from build123d import *

# Parameters (mm, degrees)
F2_DEPTH      = 20
F3_W          = 1
F3_H          = 28.1
F4_DEPTH      = 15.101
F4_DEPTH_BACK = 15.101
F5_R          = 2.6
F6_DEPTH      = 15.101
F6_DEPTH_BACK = 15.101
F7_R          = 2.6
F8_DEPTH      = 8
F9_R          = 5
F10_DEPTH     = 3
F11_S5_R      = 5
F11_T6_DEPTH  = 9
F11_S11_R     = 5
F11_T12_DEPTH = 9
F12_R         = 1


# Not quite as in the source:
# - a fillet or chamfer that OpenCascade refuses, or shapes differently, is made with other operations: its cross-section is extruded or revolved along the edge and cut away or added


with BuildPart() as f2:
    # F1 (on Front) → F2 (new body, symmetric)
    with BuildSketch(Plane.XZ):
        Polygon((15.1, 16), (10.1, 16), (10.1, -10.1), (-10.1, -10.1), (-10.1, 16), (-15.1, 16), (-15.1, -18.1), (15.1, -18.1), align=None)
    extrude(amount=F2_DEPTH, both=True)

    # F3 (on Right) → F4 (cut, two sides)
    with BuildSketch(Plane.YZ) as f4_sk:
        with Locations((0, 1.95)):
            Rectangle(F3_W, F3_H)
    extrude(amount=-F4_DEPTH, mode=Mode.SUBTRACT)
    extrude(f4_sk.sketch, amount=F4_DEPTH_BACK, mode=Mode.SUBTRACT)

    # F5 (on Right) → F6 (cut, two sides)
    with BuildSketch(Plane.YZ) as f6_sk:
        with Locations((10, 0)):
            Circle(F5_R)
        with Locations((-10, 0)):
            Circle(F5_R)
    extrude(amount=-F6_DEPTH, mode=Mode.SUBTRACT)
    extrude(f6_sk.sketch, amount=F6_DEPTH_BACK, mode=Mode.SUBTRACT)

    # F7 (on face) → F8 (cut, through all)
    with BuildSketch(Plane(origin=(0, 0, -18.1), x_dir=(1, 0, 0), z_dir=(0, 0, -1))):
        with Locations((0, 10)):
            Circle(F7_R)
        with Locations((0, -10)):
            Circle(F7_R)
    extrude(amount=-F8_DEPTH, mode=Mode.SUBTRACT)

    # F9 (on face) → F10 (cut)
    with BuildSketch(Plane(origin=(0, 0, -18.1), x_dir=(1, 0, 0), z_dir=(0, 0, -1))):
        with Locations((0, 10)):
            Circle(F9_R)
        with Locations((0, -10)):
            Circle(F9_R)
    extrude(amount=-F10_DEPTH, mode=Mode.SUBTRACT)

    # F11: chamfer of 2.5 x 1.443375673 on 2 edges, made by hand


with BuildPart() as f11_tool2:
    # F11_s3 → F11_t4 (revolve)
    with BuildSketch(Plane.XZ.offset(10)):
        Polygon((5.1, -15.1), (2.6, -13.656624327), (2.6, -15.1), align=None)
    revolve(axis=Axis((0, -10, -15.1), (0, 0, -1)))

    # F11_s5 → F11_t6 (intersect, symmetric)
    with BuildSketch(Plane.XY.offset(-14.4)):
        with Locations((0, -10)):
            Circle(F11_S5_R)
    extrude(amount=F11_T6_DEPTH, both=True, mode=Mode.INTERSECT)


with BuildPart() as f2_1:
    add(f2.part)

    # F11_t1: cut F11_tool2
    add(f11_tool2.part, mode=Mode.SUBTRACT)


with BuildPart() as f11_tool8:
    # F11_s9 → F11_t10 (revolve)
    with BuildSketch(Plane.XZ.offset(-10)):
        Polygon((2.6, -13.656624327), (5.1, -15.1), (2.6, -15.1), align=None)
    revolve(axis=Axis((0, 10, -15.1), (0, 0, -1)))

    # F11_s11 → F11_t12 (intersect, symmetric)
    with BuildSketch(Plane.XY.offset(-14.4)):
        with Locations((0, 10)):
            Circle(F11_S11_R)
    extrude(amount=F11_T12_DEPTH, both=True, mode=Mode.INTERSECT)


with BuildPart() as f2_2:
    add(f2_1.part)

    # F11_t7: cut F11_tool8
    add(f11_tool8.part, mode=Mode.SUBTRACT)

    # F12
    f12_edges = [f2_2.edges().sort_by_distance(p)[0] for p in [
        (-10.1, -10.25, -10.1),
        (-10.1, 10.25, -10.1),
        (10.1, -10.25, -10.1),
        (10.1, 10.25, -10.1),
        (-12.6, 20, 16),
        (12.6, 0.5, 16),
        (-12.6, 0.5, 16),
        (12.6, -0.5, 16),
        (-12.6, -0.5, 16),
        (-12.6, -20, 16),
        (12.6, 20, 16),
        (12.6, -20, 16),
    ]]
    fillet(f12_edges, radius=F12_R)


solid = f2_2.part
Build history of the part. All positions in model axes, mm. A direction names the side the tool comes from. Coordinates: 2 decimals unless noted, no trailing zeros. Order: outer loops, then holes, each group sorted by start corner. A loop starts at its lowest first (then second) coordinate and runs counter-clockwise, first axis right, second up. Notation, with made-up numbers: (79, 25) -> (84, 25) arc R19 ccw to (84, 44) -> close; hole circle Ø3 at (57, 66.5). An arc over 180 degrees is marked (long way). One line per item, written item: value.
(1) Slice it at C-C, the plane z = 0. Count the separate pieces of the cut face and the enclosed holes in it, plus the area to 3 significant figures.
Checked values:
separate pieces: 8
enclosed holes: 0
area: 286 mm2
(2) Slice it at A-A, the plane z = -11.5. List the corners of the cut face in (x, y).
Checked values:
outline: (-15.1, -20) -> (15.1, -20) -> (15.1, -0.5) -> (-15.1, -0.5) -> close; (-15.1, 0.5) -> (15.1, 0.5) -> (15.1, 20) -> (-15.1, 20) -> close; hole circle Ø5.2 at (0, -10); hole circle Ø5.2 at (0, 10)
(3) Probe line 1 (Y direction, x = 0, z = -12.65); line 2 (Y direction, x = 11.8, z = 0); line 3 (Y direction, x = 0, z = -16.75). List the from-to ranges inside material, lowest first. Write a range as [from, to].
Checked values:
line 1: [-20, -12.6], [-7.4, 7.4], [12.6, 20]
line 2: [-20, -12.6], [-7.4, -0.5], [0.5, 7.4], [12.6, 20]
line 3: [-20, -15], [-5, 5], [15, 20]
(4) Tool access for faces 4 (the cylindrical face through (-12.635, -0.801, 15.715)), 5 (the cylindrical face through (-0.651, -14.957, -16.593)), 6 (the cylindrical face through (12.56, -7.52, 0.78)), 7 (the cylindrical face through (9.799, -10.386, -9.815)), 8 (the cylindrical face through (-12.635, 19.715, 15.699)): list every direction of +Z, -Z, +X, -X, +Y, -Y with a clear straight run to the whole face (end or side of a thin tool).
Checked values:
face 4: +Z, +X, -X
face 5: -Z
face 6: +X, -X
face 7: +Z, +Y, -Y
face 8: +Z, +X, -X, +Y
(5) Slice it at B-B, the plane y = 10. List the corners of the cut face in (x, z).
Checked values:
outline: (-15.1, -18.1) -> (-5, -18.1) -> (-5, -15.04) -> (-2.6, -13.66) -> (-2.6, -10.1) -> (-9.1, -10.1) arc R1 cw to (-10.1, -9.1) -> (-10.1, -2.6) -> (-15.1, -2.6) -> close; (-15.1, 2.6) -> (-10.1, 2.6) -> (-10.1, 16) -> (-15.1, 16) -> close; (2.6, -13.66) -> (5, -15.04) -> (5, -18.1) -> (15.1, -18.1) -> (15.1, -2.6) -> (10.1, -2.6) -> (10.1, -9.1) arc R1 cw to (9.1, -10.1) -> (2.6, -10.1) -> close; (10.1, 2.6) -> (15.1, 2.6) -> (15.1, 16) -> (10.1, 16) -> close
(6) Drop flat-ended pins along their axis: pin 1 Ø6 at (x, y) = (0, -10) entering from +Z; pin 2 Ø13.5 at (x, z) = (-4, -5) entering from +Y; pin 3 Ø9 at (x, y) = (0, 10) entering from -Z; pin 4 Ø8 at (x, y) = (0, -10) entering from -Z. Give the stop position or say it passes through.
Checked values:
pin 1: z = -10.1
pin 2: y = 20
pin 3: z = -14.75
pin 4: z = -14.46
(7) Slice it at D-D, the plane x = 0. List the corners of the cut face in (y, z).
Checked values:
outline: (-20, -18.1) -> (-15, -18.1) -> (-15, -15.04) -> (-12.6, -13.66) -> (-12.6, -10.1) -> (-20, -10.1) -> close; (-7.4, -13.66) -> (-5, -15.04) -> (-5, -18.1) -> (5, -18.1) -> (5, -15.04) -> (7.4, -13.66) -> (7.4, -10.1) -> (0.5, -10.1) -> (0.5, -12.1) -> (-0.5, -12.1) -> (-0.5, -10.1) -> (-7.4, -10.1) -> close; (12.6, -13.66) -> (15, -15.04) -> (15, -18.1) -> (20, -18.1) -> (20, -10.1) -> (12.6, -10.1) -> close
(8) Mould opens along Y. For faces 1 (the cylindrical face through (12.565, 19.699, 15.715)), 2 (the cylindrical face through (12.635, -0.785, 15.699)), 3 (the flat face through (-13, -10, 16)) say: pulls with the +Y half, pulls with the -Y half, needs draft (parallel to the pull), parting line crosses it, or undercut.
Checked values:
face 1: pulls with the +Y half
face 2: undercut
face 3: needs draft
